Source: CAD feature listing. Evaluate the final solid. Frame: model axes, mm. Face numbers are marked on the shaded views. A direction names the side the tool comes from. Coordinates: 2 decimals unless noted, no trailing zeros. Loops run counter-clockwise (first coordinate to the right, second up) from the corner with the lowest first, then second, coordinate; pieces in that order, holes last. Notation, with made-up numbers: M 52,14 L 104,14 A18 cw 104,30 Z; hole C 45.25,-35.75 d2. An arc over 180 degrees is marked long. Write each question's results on one line, items separated by ' | '. Start each with the question number.
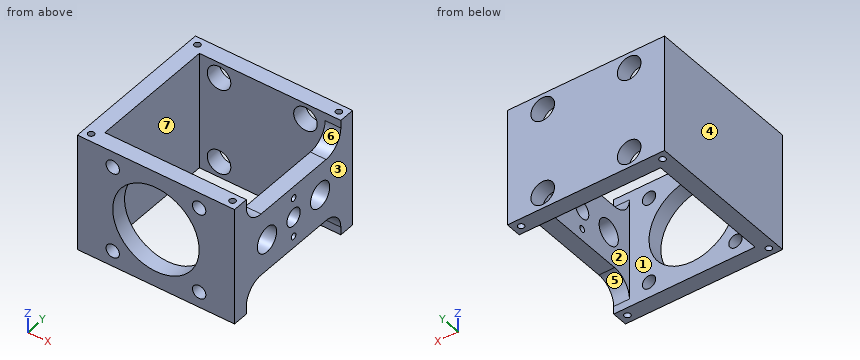
Autodesk Inventor part; units mm, degrees
ref_plane "Arbeitsebene1" through (0, 0, 15) normal (0, 0, 1) x (1, 0, 0)
ref_plane "YZ Plane" through (0, 0, 0) normal (1, 0, 0) x (0, 1, 0)
ref_plane "XZ Plane" through (0, 0, 0) normal (0, 1, 0) x (-1, 0, 0)
sketch "Skizze1" plane through (0, 0, 0) normal (0, 0, 1) x (1, 0, 0)
  line L0 (-20, 20) -> (20, 20)
  line L1 (20, 20) -> (20, -20)
  line L2 (20, -20) -> (-20, -20)
  line L3 (-20, -20) -> (-20, 20)
  line L4 (-28, 0) -> (28, 0)
  line L5 (0, -28) -> (0, 28)
  line L6 (16, 16) -> (-16, 16)
  line L7 (-16, 16) -> (-16, -16)
  line L8 (-16, -16) -> (16, -16)
  line L9 (16, -16) -> (16, 16)
  point P0 (0, 0)
  dimension "d0" = 40
  dimension "d1" = 4
extrude "Extrusion1" add sketch "Skizze1" along normal blind 30 contours L0 L5 L6 L7 L4 L3 | L0 L1 L4 L9 L6 L5 | L4 L7 L8 L5 L2 L3 | L1 L2 L5 L8 L9 L4
sketch "Skizze2" plane through (20, -20, 0) normal (1, 0, 0) x (0, 0, -1)
  line L0 (-30, 40) -> (-30, 0)
  line L1 (0, 0) -> (-30, 0)
  line L2 (0, 40) -> (-30, 40)
  line L3 (0, -8) -> (0, 48)
  line L4 (6, 20) -> (-36, 20)
  line L5 (-30, 36) -> (-28, 36)
  line L6 (-23, 31) -> (-23, 9)
  line L7 (-28, 4) -> (-30, 4)
  line L8 (-30, 4) -> (-30, 36)
  line L9 (0, 36) -> (-2, 36)
  line L10 (-7, 31) -> (-7, 9)
  line L11 (-2, 4) -> (0, 4)
  line L12 (0, 4) -> (0, 36)
  line L13 (-15, 40) -> (-15, 0)
  line L14 (0, 4) -> (-30, 4)
  arc A0 (-23, 31) -> (-28, 36) centre (-28, 31) ccw
  arc A1 (-28, 4) -> (-23, 9) centre (-28, 9) ccw
  arc A2 (-7, 9) -> (-2, 4) centre (-2, 9) ccw
  arc A3 (-2, 36) -> (-7, 31) centre (-2, 31) ccw
  point P0 (0, 20)
  dimension "d5" = 16
  dimension "d6" = 5
extrude "Extrusion2" cut sketch "Skizze2" against normal up to surface (4 mm away) contours L5 A0 L6 L4 L0 | L4 L6 A1 L7 L0 | L3 L4 L10 A3 L9 | L4 L3 L11 A2 L10
sketch "Skizze4" plane through (20, -20, 0) normal (1, 0, 0) x (0, 0, -1)
  circle A0 centre (-20, 20) radius 1.15
  circle A1 centre (-10, 20) radius 1.15
  point P0 (0, 20)
hole "Bohrung2" at (20, 0, 20) at (20, 0, 10) direction (-1, 0, 0) diameter 1.567 end up to surface
sketch "Skizze5" plane through (20, -20, 0) normal (1, 0, 0) x (0, 0, -1)
  circle A0 centre (-15, 20) radius 2
  point P0 (0, 20)
hole "Bohrung3" at (20, 0, 15) direction (-1, 0, 0) diameter 4.5 end up to surface
sketch "Skizze6" plane through (-20, -20, 0) normal (0, -1, 0) x (1, 0, 0)
  line L0 (40, 30) -> (0, 30)
  line L1 (0, 0) -> (0, 30)
  line L2 (40, 0) -> (40, 30)
  line L3 (40, 15) -> (0, 15)
  line L4 (20, 0) -> (20, 30)
  point P0 (20, 15)
hole "Bohrung4" at (0, -20, 15) direction (0, 1, 0) diameter 22 end up to surface
sketch "Skizze7" plane through (20, -20, 0) normal (1, 0, 0) x (0, 0, -1)
  line L0 (0, 0) -> (-30, 0)
  line L1 (-7, 9) -> (-7, 31)
  line L2 (0, 40) -> (-30, 40)
  line L3 (-23, 31) -> (-23, 9)
  line L4 (-15, 0) -> (-15, 40)
  line L5 (-23, 20) -> (-7, 20)
  point P0 (0, 20)
  point P1 (-15, 11)
  point P2 (-15, 29)
  dimension "d43" = 18
hole "Bohrung5" at (20, -9, 15) at (20, 9, 15) direction (-1, 0, 0) diameter 6.5 end up to surface
sketch "Skizze8" plane through (-20, -20, 0) normal (0, -1, 0) x (1, 0, 0)
  circle A0 centre (20, 15) radius 11
  line L0 (9, 26) -> (31, 26)
  line L1 (31, 26) -> (31, 4)
  line L2 (31, 4) -> (9, 4)
  line L3 (9, 4) -> (9, 26)
  line L4 (-8, 0) -> (48, 0)
  line L5 (20, -6) -> (20, 36)
  line L6 (20, 15) -> (29.164, 15)
  point P0 (20, 0)
  dimension "d51" = 22
hole "Bohrung6" at (-11, -20, 26) at (11, -20, 26) at (11, -20, 4) at (-11, -20, 4) direction (0, 1, 0) diameter 3.4 end through all
sketch "Skizze9" plane through (-20, 20, 0) normal (0, 1, 0) x (1, 0, 0)
  circle A0 centre (9, -4) radius 1.7
  circle A1 centre (31, -4) radius 1.7
  circle A2 centre (31, -26) radius 1.7
  circle A3 centre (9, -26) radius 1.7
  point P0 (20, 0)
hole "Bohrung7" at (-11, 20, 4) at (11, 20, 4) at (11, 20, 26) at (-11, 20, 26) direction (0, -1, 0) diameter 6 depth 8 tip angle 118
sketch "Skizze10" plane through (0, 0, 30) normal (0, 0, 1) x (1, 0, 0)
  line L0 (20, 20) -> (20, 16)
  line L1 (-20, 20) -> (20, 20)
  line L2 (-20, -20) -> (-20, 20)
  line L3 (20, -20) -> (-20, -20)
  line L4 (-18, 18) -> (18, 18)
  line L5 (18, 18) -> (18, -18)
  line L6 (18, -18) -> (-18, -18)
  line L7 (-18, -18) -> (-18, 18)
  point P0 (0, 0)
  dimension "d66" = 2
  dimension "d67" = 2
  dimension "d68" = 2
  dimension "d69" = 2
hole "Bohrung8" at (-18, 18, 30) at (18, 18, 30) at (18, -18, 30) at (-18, -18, 30) direction (0, 0, -1) diameter 1.567 depth 8 tip angle 118
ref_plane "Arbeitsebene1" through (0, 0, 15) normal (0, 0, 1) x (1, 0, 0)
mirror "Spiegeln1" about plane through (0, 0, 15) normal (0, 0, 1) of "Bohrung8"
properties part number "13_0204_016"
Item 1: First-contact query: pin 1 Ø4.5 at (x, y) = (19, -4.5) entering from +Z; pin 2 Ø4 at (x, z) = (-5.5, 9) entering from -Y; pin 3 Ø4 at (x, y) = (15.5, -13) entering from -Z. Flat tips, straight axial feed; report the tip coordinate or a pass-through.
Item 2: Cut plane A-A (y = -9). Output: boundary loops of the cut face in (x, z), then the cut area to 3 significant figures.
Item 3: Line query: probe 1 along Y at (x, z) = (-18, 5.75); probe 2 along Y at (x, z) = (18, 2); probe 3 along Z at (x, y) = (11, 17). Output: solid intervals per line, ascending.
Item 4: Cut plane B-B (x = 0). Output: boundary loops of the cut face in (y, z).
Item 5: Cut plane C-C (y = 14). Output: boundary loops of the cut face in (x, z).
Item 6: Cut plane D-D (z = 20). Output: boundary loops of the cut face in (x, y), then the cut area to 3 significant figures.
Item 7: Mould query, pull axis X, two halves, no side actions, for the marked faces 1, 2, 3 and 4. Classes: +X half, -X half, draft (parallel to the pull), parting line (faces both ways), or undercut.
Item 8: Access query for the marked faces 5, 6 and 7. Directions: +Z, -Z, +X, -X, +Y, -Y. A direction counts if a zero-diameter tool reaches every point of the face in a straight line with its end or side. Return the directions, or none.
Response values:
1) pin 1: stops at z = 23 | pin 2: stops at y = 16 | pin 3: stops at z = 5.08
2) outline: M -20,0 L -16,0 L -16,30 L -20,30 Z; M 16,7 L 20,7 L 20,11.75 L 16,11.75 Z; M 16,18.25 L 20,18.25 L 20,23 L 16,23 Z | area: 158 mm2
3) probe 1: y = -20 to -18.78, -17.22 to 17.22, 18.78 to 20 | probe 2: y = -20 to -18.78, -17.22 to -16, 16 to 17.22, 18.78 to 20 | probe 3: z = 0 to 1, 7 to 23, 29 to 30
4) outline: M -20,0 L -16,0 L -16,4 L -20,4 Z; M -20,26 L -16,26 L -16,30 L -20,30 Z; M 16,0 L 20,0 L 20,30 L 16,30 Z
5) outline: M -20,0 L -16,0 L -16,30 L -20,30 Z; M 16,6 L 20,6 L 20,24 L 16,24 Z
6) outline: M -20,-20 L -9.8,-20 L -9.8,-16 L -16,-16 L -16,16 L 16,16 L 16,0.78 L 20,0.78 L 20,20 L -20,20 Z; M 9.8,-20 L 20,-20 L 20,-0.78 L 16,-0.78 L 16,-16 L 9.8,-16 Z | area: 491 mm2
7) face 1: undercut | face 2: undercut | face 3: +X half | face 4: -X half
8) face 5: -Z, +X | face 6: +Z, +X | face 7: +Z, -Z
